```python
from build123d import *

# Parameters (mm, degrees)
SKETCH2_R           = 8.75
BOSS_EXTRUDE1_DEPTH = 14
SKETCH3_R           = 1.4
BOSS_EXTRUDE2_DEPTH = 3
FILLET1_R           = 1
CUT_EXTRUDE2_REACH  = 49.033


with BuildPart() as part:
    # Sketch2 → Boss-Extrude1 (new body)
    with BuildSketch(Plane.XY):
        Circle(SKETCH2_R)
    extrude(amount=BOSS_EXTRUDE1_DEPTH)

    # Sketch3 → Boss-Extrude2 (add)
    with BuildSketch(Plane.XY):
        with BuildLine():
            ThreePointArc((-12.038357667, -12.701493797), (-12.374368671, -12.374368671), (-12.701493797, -12.038357667))
            ThreePointArc((-12.701493797, -12.038357667), (-18.306346632, -8.128131702), (-25, -6.75))
            ThreePointArc((-25, -6.75), (-31.75, 0), (-25, 6.75))
            ThreePointArc((-25, 6.75), (-18.306346632, 8.128131702), (-12.701493797, 12.038357667))
            ThreePointArc((-12.701493797, 12.038357667), (-12.374368671, 12.374368671), (-12.038357667, 12.701493797))
            ThreePointArc((-12.038357667, 12.701493797), (-8.128131702, 18.306346632), (-6.75, 25))
            ThreePointArc((-6.75, 25), (0, 31.75), (6.75, 25))
            ThreePointArc((6.75, 25), (8.128131702, 18.306346632), (12.038357667, 12.701493797))
            ThreePointArc((12.038357667, 12.701493797), (12.374368671, 12.374368671), (12.701493797, 12.038357667))
            ThreePointArc((12.701493797, 12.038357667), (18.306346632, 8.128131702), (25, 6.75))
            ThreePointArc((25, 6.75), (31.75, 0), (25, -6.75))
            ThreePointArc((25, -6.75), (18.306346632, -8.128131702), (12.701493797, -12.038357667))
            ThreePointArc((12.701493797, -12.038357667), (12.374368671, -12.374368671), (12.038357667, -12.701493797))
            ThreePointArc((12.038357667, -12.701493797), (8.128131702, -18.306346632), (6.75, -25))
            ThreePointArc((6.75, -25), (0, -31.75), (-6.75, -25))
            ThreePointArc((-6.75, -25), (-8.128131702, -18.306346632), (-12.038357667, -12.701493797))
        make_face()
        with Locations((25, 0)):
            Circle(SKETCH3_R, mode=Mode.SUBTRACT)
        with Locations((0, -25)):
            Circle(SKETCH3_R, mode=Mode.SUBTRACT)
        with Locations((-25, 0)):
            Circle(SKETCH3_R, mode=Mode.SUBTRACT)
        with Locations((0, 25)):
            Circle(SKETCH3_R, mode=Mode.SUBTRACT)
    extrude(amount=BOSS_EXTRUDE2_DEPTH)

    # Fillet1
    fillet1_edges = [part.edges().sort_by_distance(p)[0] for p in [
        (-8.75, 0, 14),
        (-8.75, 0, 3),
    ]]
    fillet(fillet1_edges, radius=FILLET1_R)

    # Sketch1 → Cut-Extrude2 (cut, up to next)
    with BuildSketch(Plane.XY, mode=Mode.PRIVATE) as cut_extrude2_sk1:
        Polygon((2.612789059, -2.612789059), (3.569136229, 0.95634717), (0.95634717, 3.569136229), (-2.612789059, 2.612789059), (-3.569136229, -0.95634717), (-0.95634717, -3.569136229), align=None)
    cut_extrude2_tool1 = extrude(cut_extrude2_sk1.sketch, amount=CUT_EXTRUDE2_REACH, mode=Mode.PRIVATE) & part.part
    add(cut_extrude2_tool1.solids().sort_by_distance((0, 0, 0))[0], mode=Mode.SUBTRACT)


solid = part.part
```
CAD build for the part. Positions are in the model's coordinates, mm. A direction names the side the tool comes from. Coordinates: 2 decimals unless noted, no trailing zeros. Order: outer loops, then holes, each group sorted by start corner. A loop starts at its lowest first (then second) coordinate and runs counter-clockwise, first axis right, second up. Notation, with made-up numbers: (5.25, 63.5) -> (58.25, 63.5) arc R25 ccw to (58.25, 89.5) -> close; hole circle Ø6 at (0.25, -25). An arc over 180 degrees is marked (long way). Use one line per item in the form item = value. Start each with the question number.
1) Drop flat-ended pins along their axis: pin 1 (5 mm diameter, centred on y = -25, z = 3.5, fed in from +X); pin 2 (1 mm diameter, centred on y = 18.5, z = 1.5, fed in from +X); pin 3 (5 mm diameter, centred on x = 10.5, y = -18.5, fed in from +Z). Give the stop position or say it passes through.
2) Band-saw the part on C-C on y = 0. Give the cut face in (x, z), then the cut area to 3 significant figures.
3) Tool access for faces 4 (the flat face through (3, -2, 14)), 5 (the flat face through (0.8, -3.1, 6.9)), 6 (the cylindrical face through (-6.944, -5.324, 8.437)): list every direction of +Z, -Z, +X, -X, +Y, -Y with a clear straight run to the whole face (end or side of a thin tool).
4) Band-saw the part on D-D on x = 14. Give the cut face in (y, z), then the cut area to 3 significant figures.
5) Drill centre lines: L1, parallel to Y at x = 0, z = 1.7; L2, parallel to Y at x = 25, z = 1.3. Where is each one in solid material? Low to high. Write a range as [from, to].
6) Pull direction Y, two halves, no side cores. Call faces 1 (the flat face through (0, -7, 0)), 2 (the cylindrical face through (-0.303, -26.367, 1.479)), 3 (the cylindrical face through (-8.09, -18.395, 1.479)): +Y half, -Y half, draft (parallel to the pull), parting line (faces both ways), or undercut.
7) Band-saw the part on B-B on z = 6.75. Give the cut face in (x, y).
8) Band-saw the part on A-A on z = 2.25. Give the cut face in (x, y).
Entries:
q1.pin_1 = 6.93
q1.pin_2 = 8.26
q1.pin_3 = 3
q2.outline = (-31.75, 0) -> (-26.4, 0) -> (-26.4, 3) -> (-31.75, 3) -> close; (-23.6, 0) -> (-3.31, 0) -> (-3.31, 14) -> (-7.75, 14) arc R1 ccw to (-8.75, 13) -> (-8.75, 4) arc R1 cw to (-9.75, 3) -> (-23.6, 3) -> close; (3.31, 0) -> (23.6, 0) -> (23.6, 3) -> (9.75, 3) arc R1 cw to (8.75, 4) -> (8.75, 13) arc R1 ccw to (7.75, 14) -> (3.31, 14) -> close; (26.4, 0) -> (31.75, 0) -> (31.75, 3) -> (26.4, 3) -> close
q2.area = 273 mm2
q3.face_4 = +Z, +X, -X, +Y, -Y
q3.face_5 = +Z, -Z
q3.face_6 = +Z
q4.outline = (-10.81, 0) -> (10.81, 0) -> (10.81, 3) -> (-10.81, 3) -> close
q4.area = 64.8 mm2
q5.L1 = [-31.75, -26.4], [-23.6, -3.31], [3.31, 23.6], [26.4, 31.75]
q5.L2 = [-6.75, -1.4], [1.4, 6.75]
q6.face_1 = draft
q6.face_2 = undercut
q6.face_3 = -Y half
q7.outline = circle Ø17.5 at (0, 0); hole (-3.57, -0.96) -> (-0.96, -3.57) -> (2.61, -2.61) -> (3.57, 0.96) -> (0.96, 3.57) -> (-2.61, 2.61) -> close
q8.outline = (-25, -6.75) arc R16.94 cw to (-12.7, -12.04) arc R17.5 ccw to (-12.04, -12.7) arc R16.94 cw to (-6.75, -25) arc R6.75 ccw to (6.75, -25) arc R16.94 cw to (12.04, -12.7) arc R17.5 ccw to (12.7, -12.04) arc R16.94 cw to (25, -6.75) arc R6.75 ccw to (25, 6.75) arc R16.94 cw to (12.7, 12.04) arc R17.5 ccw to (12.04, 12.7) arc R16.94 cw to (6.75, 25) arc R6.75 ccw to (-6.75, 25) arc R16.94 cw to (-12.04, 12.7) arc R17.5 ccw to (-12.7, 12.04) arc R16.94 cw to (-25, 6.75) arc R6.75 ccw to start; hole circle Ø2.8 at (-25, 0); hole (-3.57, -0.96) -> (-0.96, -3.57) -> (2.61, -2.61) -> (3.57, 0.96) -> (0.96, 3.57) -> (-2.61, 2.61) -> close; hole circle Ø2.8 at (0, -25); hole circle Ø2.8 at (0, 25); hole circle Ø2.8 at (25, 0)
